Here's the drawing with two shaded views (mm, measured from the low corner). I have some questions. A direction names the side the tool comes from. Coordinates: 2 decimals unless noted, no trailing zeros. Write each loop counter-clockwise with the first axis right and the second up, starting at its lowest first coordinate (ties: lowest second). Pieces come first, ordered by that corner, then holes. Notation, with made-up numbers: M 71,10.5 L 81,10.5 A10 ccw 81,16.5 Z; hole C 34.25,-20 d11. An arc over 180 degrees is marked long. Use one line per item in the form item = value. Start each with the question number.
1. I want a section at A-A, the plane y = 13.5. List the corners of the cut face in (x, z) for me.
2. I want a section at B-B, the plane x = 87. List the corners of the cut face in (y, z) for me.
3. On a 3-axis mill with a long thin cutter (end or side, diameter ignored), from which of +Z, -Z, +X, -X, +Y, -Y can I reach the whole of each face in a straight line? I mean the marked faces 1 and 2. Say none if no direction works.
4. I'm going to push flat-ended pins straight in: pin 1 Ø15 at (y, z) = (7.5, 52.5) entering from +X; pin 2 Ø21 at (x, y) = (107, 8.5) entering from +Z; pin 3 Ø4 at (x, z) = (109.5, 37.5) entering from -Y. Where does each tip first touch, or does it pass through?
5. Please list where these lines run through material, in increasing order: line 1 along Z through (x, y) = (76, 11); line 2 along Y through (x, z) = (96, 37); line 3 along X through (y, z) = (10, 58). Write a range as [from, to].
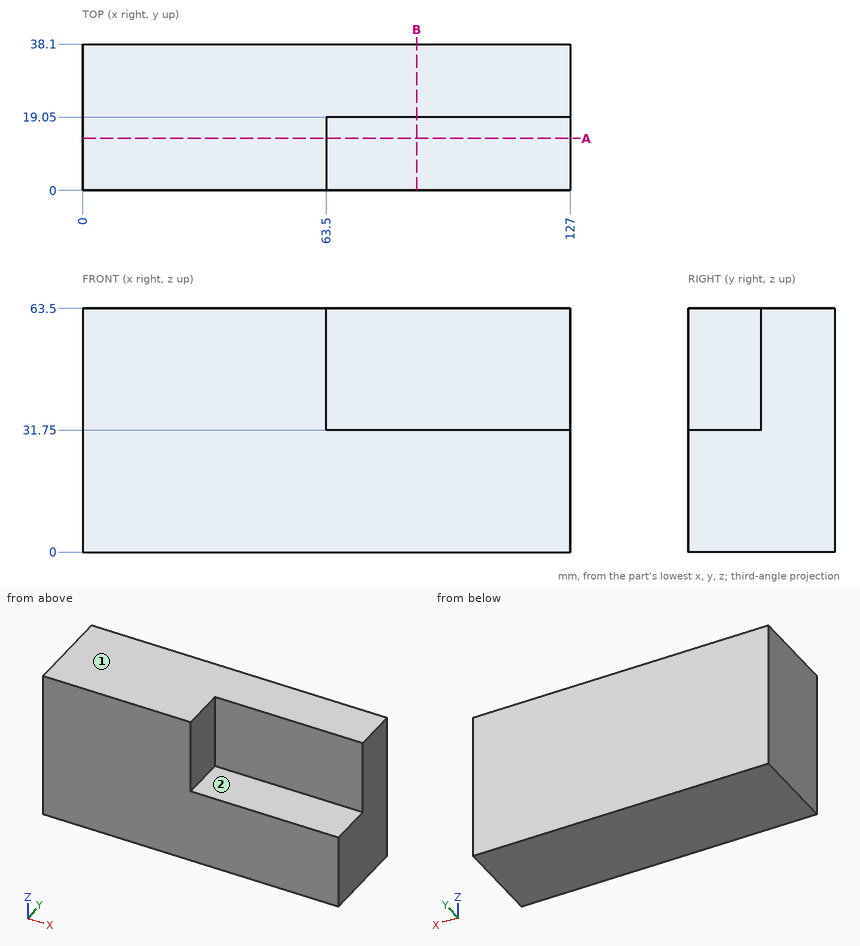
Answer list:
q1.outline = M 0,0 L 127,0 L 127,31.75 L 63.5,31.75 L 63.5,63.5 L 0,63.5 Z
q2.outline = M 0,0 L 38.1,0 L 38.1,63.5 L 19.05,63.5 L 19.05,31.75 L 0,31.75 Z
q3.face_1 = +Z, +X, -X, +Y, -Y
q3.face_2 = +Z, +X, -Y
q4.pin_1 = 63.5
q4.pin_2 = 31.75
q4.pin_3 = 19.05
q5.line_1 = [0, 31.75]
q5.line_2 = [19.05, 38.1]
q5.line_3 = [0, 63.5]
